Geometry check sheet. Reference: the model listing, model coordinates, mm. A direction names the side the tool comes from. Coordinates: 2 decimals unless noted, no trailing zeros. Write each loop counter-clockwise with the first axis right and the second up, starting at its lowest first coordinate (ties: lowest second). Pieces come first, ordered by that corner, then holes. Notation, with made-up numbers: (-15, 64.5) -> (33, 64.5) arc R7 ccw to (33, 68.5) -> close; hole circle Ø7 at (24.5, 2). An arc over 180 degrees is marked (long way). One line per question, with ' | ' between items.
from build123d import *

# Parameters (mm, degrees)
F1_DEPTH = 20
F3_D     = 8.8
F5_D     = 4.4


with BuildPart() as f1:
    # F0 (on Top) → F1 (new body)
    with BuildSketch(Plane.XY):
        with BuildLine():
            Line((0, 70), (0, 0))
            Line((0, 0), (2, 0))
            Line((2, 0), (2, 70))
            ThreePointArc((2, 70), (4.3431457505, 75.6568542495), (10, 78))
            Line((10, 78), (46, 78))
            ThreePointArc((46, 78), (51.6568542495, 75.6568542495), (54, 70))
            Line((54, 70), (54, 0))
            Line((54, 0), (56, 0))
            Line((56, 0), (56, 70))
            ThreePointArc((56, 70), (53.0710678119, 77.0710678119), (46, 80))
            Line((46, 80), (10, 80))
            ThreePointArc((10, 80), (2.9289321881, 77.0710678119), (0, 70))
        make_face()
    extrude(amount=F1_DEPTH)

    # F3 (through all)
    with Locations(Plane.YZ.offset(56)):
        with Locations((55, 10)):
            Hole(F3_D / 2)

    # F5 (through all)
    with Locations(Plane.YZ.offset(56)):
        with Locations((5, 10), (20, 10)):
            Hole(F5_D / 2)


solid = f1.part
1. Cross-section at C-C on z = 10. Give the number of separate pieces and of enclosed holes in the cut face, and give its area (3 significant figures).
Worked answers:
separate pieces: 7 | enclosed holes: 0 | area: 338 mm²
2. Cross-section at A-A on y = 12.5. Record the boundary of the cut face in (x, z), and give its area (3 significant figures).
Worked answers:
outline: (0, 0) -> (2, 0) -> (2, 20) -> (0, 20) -> close; (54, 0) -> (56, 0) -> (56, 20) -> (54, 20) -> close | area: 80.0 mm²
3. Cross-section at B-B on y = 55. Record the boundary of the cut face in (x, z).
Worked answers:
outline: (0, 0) -> (2, 0) -> (2, 5.6) -> (0, 5.6) -> close; (0, 14.4) -> (2, 14.4) -> (2, 20) -> (0, 20) -> close; (54, 0) -> (56, 0) -> (56, 5.6) -> (54, 5.6) -> close; (54, 14.4) -> (56, 14.4) -> (56, 20) -> (54, 20) -> close
4. Go/stop test with flat-tipped pins: P1, Ø12, axis at x = 7.5, y = 26.5, coming from the +Z side; P2, Ø6, axis at x = 21, z = 5.5, coming from the -Y side. Record where each tip stops, or that it passes through.
Worked answers:
P1: z = 20 | P2: y = 78
5. Cross-section at D-D on z = 15.5. Record the boundary of the cut face in (x, y).
Worked answers:
outline: (0, 0) -> (2, 0) -> (2, 70) arc R8 cw to (10, 78) -> (46, 78) arc R8 cw to (54, 70) -> (54, 0) -> (56, 0) -> (56, 70) arc R10 ccw to (46, 80) -> (10, 80) arc R10 ccw to (0, 70) -> close
6. Material ranges on line 1 (Z direction, x = 55.3, y = 55); line 2 (X direction, y = 40, z = 7.5); line 3 (Y direction, x = 30.5, z = 19), recorded low to high. Write a range as from..to.
Worked answers:
line 1: 0..5.6, 14.4..20 | line 2: 0..2, 54..56 | line 3: 78..80
7. Mould release check, pull along X, two halves, no side actions. Record for faces 1 (the face through (51.594, 75.719, 9.86)), 2 (the face through (3.01, 77.15, 9.86)), 3 (the face through (0.99, 2.9, 10.66)): released by +X, released by -X, zero draft, split by the parting line, or undercut.
Worked answers:
face 1: undercut | face 2: released by -X | face 3: zero draft
8. Tool access check on faces 4 (the face through (28, 80, 10)), 5 (the face through (28, 78, 10)). Record the directions out of +Z, -Z, +X, -X, +Y, -Y that give a thin tool (end or side, any length) a straight path to the whole face; none if there is none.
Worked answers:
face 4: +Z, -Z, +X, -X, +Y | face 5: +Z, -Z, -Y
